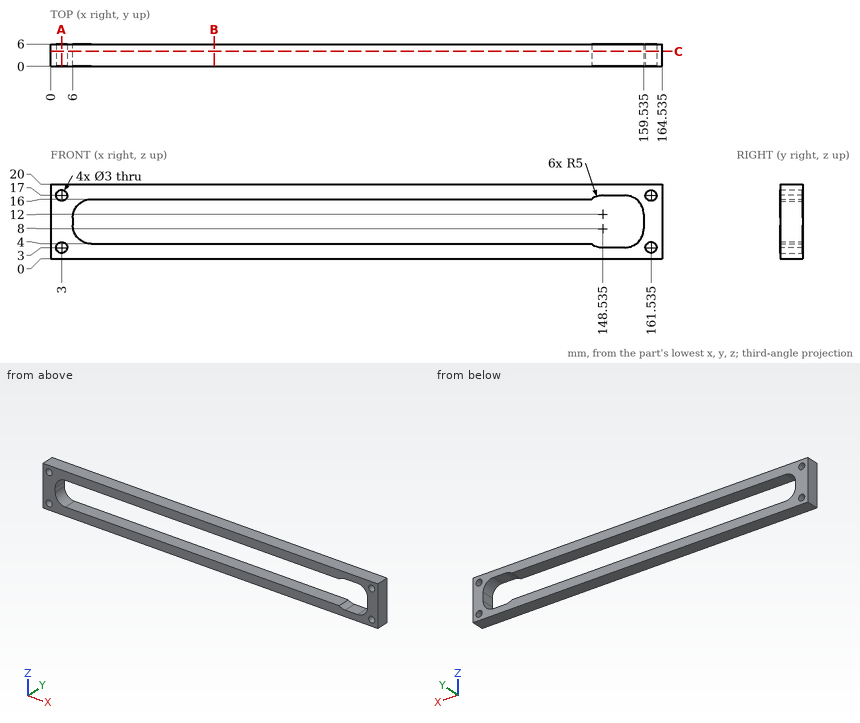
Could you check a few things on this drawing? It's one solid part, dimensions in mm from its lowest x, y, z. Round coordinates to 2 decimals unless told otherwise and drop trailing zeros. Write each loop counter-clockwise with the first axis right and the second up, starting at its lowest first coordinate (ties: lowest second). Pieces come first, ordered by that corner, then holes.
Q1. Will this pin go through, and if not, where does the flat tip stop? P1, Ø1.8, axis at x = 3, z = 17, coming from the -Y side.
Q2. If we section it at B-B on x = 44: Write out the boundary of the cut face in (y, z), plus the area to 3 significant figures.
Q3. If we section it at A-A on x = 3: Write out the boundary of the cut face in (y, z), plus the area to 3 significant figures.
Q4. If we section it at C-C on y = 4: Write out the boundary of the cut face in (x, z) (1 decimal), plus the area to 3 significant figures.
Q5. Please list where these lines run through material, in increasing order: probe 1 along Z at (x, y) = (45, 1.9); probe 2 along X at (y, z) = (1.25, 10) (1 decimal); probe 3 along Z at (x, y) = (148.5, 5.35).
Answer below:
1. P1: passes through
2. outline: (0, 0) - (6, 0) - (6, 4) - (0, 4) - close; (0, 16) - (6, 16) - (6, 20) - (0, 20) - close
2. area: 48.0 mm2
3. outline: (0, 0) - (6, 0) - (6, 1.5) - (0, 1.5) - close; (0, 4.5) - (6, 4.5) - (6, 15.5) - (0, 15.5) - close; (0, 18.5) - (6, 18.5) - (6, 20) - (0, 20) - close
3. area: 84.0 mm2
4. outline: (0, 0) - (164.5, 0) - (164.5, 20) - (0, 20) - close; hole circle Ø3 at (3, 3); hole circle Ø3 at (3, 17); hole (6, 9) arc R5 ccw to (11, 4) - (145.5, 4) arc R5 ccw to (148.5, 3) - (154.5, 3) arc R5 ccw to (159.5, 8) - (159.5, 12) arc R5 ccw to (154.5, 17) - (148.5, 17) arc R5 ccw to (145.5, 16) - (11, 16) arc R5 ccw to (6, 11) - close; hole circle Ø3 at (161.5, 3); hole circle Ø3 at (161.5, 17)
4. area: 1,420 mm2
5. probe 1: z = 0 to 4, 16 to 20
5. probe 2: x = 0 to 6, 159.5 to 164.5
5. probe 3: z = 0 to 3, 17 to 20
